```python
from build123d import *

# Parameters (mm, degrees)
BOSS_EXTRUDE2_DEPTH = 18
SKETCH4_W           = 53
SKETCH4_H           = 12
CUT_EXTRUDE2_DEPTH  = 25.4
SKETCH5_W           = 14
SKETCH5_H           = 14
CUT_EXTRUDE3_DEPTH  = 7


with BuildPart() as part:
    # Sketch3 → Boss-Extrude2 (new body)
    with BuildSketch(Plane.XY):
        Polygon((0, 0), (0, 25.4), (-11.5, 25.4), (-11.5, 32.4), (68.5, 32.4), (68.5, 25.4), (57, 25.4), (57, 0), align=None)
    extrude(amount=BOSS_EXTRUDE2_DEPTH)

    # Sketch4 → Cut-Extrude2 (cut)
    with BuildSketch(Plane.XZ):
        with Locations((28.5, 9)):
            Rectangle(SKETCH4_W, SKETCH4_H)
    extrude(amount=-CUT_EXTRUDE2_DEPTH, mode=Mode.SUBTRACT)

    # Sketch5 → Cut-Extrude3 (cut)
    with BuildSketch(Plane(origin=(0, 32.4, 0), x_dir=(1, 0, 0), z_dir=(0, 1, 0))):
        with Locations((28.5, -9)):
            Rectangle(SKETCH5_W, SKETCH5_H)
    extrude(amount=-CUT_EXTRUDE3_DEPTH, mode=Mode.SUBTRACT)


solid = part.part
```
Here's how the part is built. I have some questions about the finished solid (model axes, mm). A direction names the side the tool comes from. Give positions to 0.01 mm unless a question says otherwise; leave off trailing zeros. Write each loop counter-clockwise with the first axis right and the second up, starting at its lowest first coordinate (ties: lowest second). Pieces come first, ordered by that corner, then holes. Notation, with made-up numbers: M -4,76 L 51,76 A33 cw 51,109 Z; hole C 60,-39.5 d7. An arc over 180 degrees is marked long. Put each result on its own line as item: value. Start each with the question number.
Item 1: Thinking about a two-plate mould opening in Z: for faces 6 (the flat face through (-6, 25.4, 9)), 7 (the flat face through (2, 13, 9)), 8 (the flat face through (29, 16, 0)), 9 (the flat face through (28, 29, 2)), which applies, +Z half, -Z half, draft (parallel to the pull), parting line (faces both ways), or undercut?
Item 2: If we section it at C-C, the plane y = 29.5: Write out the boundary of the cut face in (x, z).
Item 3: If we section it at B-B, the plane z = 13.75: Write out the boundary of the cut face in (x, y).
Item 4: If we section it at D-D, the plane x = 53: Write out the boundary of the cut face in (y, z).
Item 5: Will these pins go through, and if not, where does the flat tip stop? pin 1 (0.5 mm diameter, centred on x = 31.5, z = 15.5, fed in from +Y); pin 2 (9.5 mm diameter, centred on y = 14, z = 7.5, fed in from +X); pin 3 (9.5 mm diameter, centred on y = 7, z = 9, fed in from -X); pin 4 (5 mm diameter, centred on x = 60, y = 6, fed in from +Z).
Item 6: I need wall thicknesses on L1, parallel to X at y = 31.5, z = 8.5; L2, parallel to Z at x = 37, y = 11; L3, parallel to X at y = 22, z = 12.25. Which ranges of each line are inside material? Lowest first, please. Write a range as from..to.
Item 7: On a 3-axis mill with a long thin cutter (end or side, diameter ignored), from which of +Z, -Z, +X, -X, +Y, -Y can I reach the whole of each face in a straight line? I mean faces 1 (the flat face through (21.5, 29, 9)), 2 (the flat face through (45, 25.4, 9)), 3 (the flat face through (63, 25.4, 9)), 4 (the flat face through (28, 32.4, 17)), 5 (the flat face through (0, 13, 9)). Say none if no direction works.
Item 8: If we section it at A-A, the plane x = 25: Write out the boundary of the cut face in (y, z), then the cut area to 3 significant figures.
Values:
1. face 6: draft
1. face 7: undercut
1. face 8: -Z half
1. face 9: undercut
2. outline: M -11.5,0 L 68.5,0 L 68.5,18 L -11.5,18 Z; hole M 21.5,2 L 35.5,2 L 35.5,16 L 21.5,16 Z
3. outline: M -11.5,25.4 L 0,25.4 L 0,0 L 2,0 L 2,25.4 L 21.5,25.4 L 21.5,32.4 L -11.5,32.4 Z; M 35.5,25.4 L 55,25.4 L 55,0 L 57,0 L 57,25.4 L 68.5,25.4 L 68.5,32.4 L 35.5,32.4 Z
4. outline: M 0,0 L 32.4,0 L 32.4,18 L 0,18 L 0,15 L 25.4,15 L 25.4,3 L 0,3 Z
5. pin 1: y = 25.4
5. pin 2: x = 57
5. pin 3: x = 0
5. pin 4: through
6. L1: -11.5..21.5, 35.5..68.5
6. L2: 0..3, 15..18
6. L3: 0..2, 55..57
7. face 1: +Y
7. face 2: -Y
7. face 3: +Z, -Z, +X, -Y
7. face 4: +Z, -Z, +X, -X, +Y
7. face 5: +Z, -Z, -X, -Y
8. outline: M 0,0 L 32.4,0 L 32.4,2 L 25.4,2 L 25.4,3 L 0,3 Z; M 0,15 L 25.4,15 L 25.4,16 L 32.4,16 L 32.4,18 L 0,18 Z
8. area: 180 mm²
